Verification items for the finished model (mm, model axes). Give positions to 0.01 mm unless a question says otherwise; leave off trailing zeros. Loops run counter-clockwise (first coordinate to the right, second up) from the corner with the lowest first, then second, coordinate; pieces in that order, holes last. Notation, with made-up numbers: M 28.25,74.25 L 33.25,74.25 A24 ccw 33.25,85.25 Z; hole C 44.5,-11.5 d7. An arc over 180 degrees is marked long. Answer in a Markdown table with one row per item.
```python
from build123d import *

# Parameters (mm, degrees)
F0_W     = 127
F0_H     = 127
F1_DEPTH = 127
F2_R     = 38.1
F3_DEPTH = 127.001
F4_R     = 38.1
F5_DEPTH = 127.001
F6_R     = 38.1
F7_DEPTH = 127.001


with BuildPart() as f1:
    # F0 (on Top) → F1 (new body)
    with BuildSketch(Plane.XY):
        with Locations((63.5, 63.5)):
            Rectangle(F0_W, F0_H)
    extrude(amount=F1_DEPTH)

    # F2 (on face) → F3 (cut, through all)
    with BuildSketch(Plane.XZ):
        with Locations((63.5, 63.5)):
            Circle(F2_R)
    extrude(amount=-F3_DEPTH, mode=Mode.SUBTRACT)

    # F4 (on face) → F5 (cut, through all)
    with BuildSketch(Plane.YZ.offset(127)):
        with Locations((63.5, 63.5)):
            Circle(F4_R)
    extrude(amount=-F5_DEPTH, mode=Mode.SUBTRACT)

    # F6 (on face) → F7 (cut, through all)
    with BuildSketch(Plane.XY.offset(127)):
        with Locations((63.5, 63.5)):
            Circle(F6_R)
    extrude(amount=-F7_DEPTH, mode=Mode.SUBTRACT)


solid = f1.part
```
Item 1: Scan line: L1, parallel to Z at x = 63, y = 113. Record every from-to range of solid material in increasing order. Write a range as [from, to].
Reported:
| item | result |
|---|---|
| L1 | z = [0, 25.4], [101.6, 127] |
Item 2: Sectioned sample at C-C (x = 9.5). Record the cut outline in (y, z), and give its area (3 significant figures).
Reported:
| item | result |
|---|---|
| outline | M 0,0 L 127,0 L 127,127 L 0,127 Z; hole C 63.5,63.5 d76.2 |
| area | 11,600 mm^2 |
Item 3: Sectioned sample at A-A (y = 63.5). Record the cut outline in (x, z).
Reported:
| item | result |
|---|---|
| outline | M 0,0 L 25.4,0 L 25.4,25.4 L 0,25.4 Z; M 0,101.6 L 25.4,101.6 L 25.4,127 L 0,127 Z; M 101.6,0 L 127,0 L 127,25.4 L 101.6,25.4 Z; M 101.6,101.6 L 127,101.6 L 127,127 L 101.6,127 Z |
Item 4: Release check for a two-part mould opening along X. For faces 1 (the cylindrical face through (35.42, 13.96, 89.25)), 2 (the flat face through (0, 34, 91)), 3 (the flat face through (34, 0, 91)) record: released by +X, released by -X, zero draft, split by the parting line, or undercut.
Reported:
| item | result |
|---|---|
| face 1 | undercut |
| face 2 | released by -X |
| face 3 | zero draft |
